from build123d import *

# Parameters (mm, degrees)
SKETCH1_W           = 100
SKETCH1_H           = 100
BOSS_EXTRUDE1_DEPTH = 2
BOSS_EXTRUDE2_DEPTH = 1
BOSS_EXTRUDE5_DEPTH = 1
SKETCH10_R          = 14.102334265
CUT_EXTRUDE1_DEPTH  = 1.5


with BuildPart() as part:
    # Sketch1 → Boss-Extrude1 (new body)
    with BuildSketch(Plane(origin=(0, 0, 0), x_dir=(1, 0, 0), z_dir=(0, 1, 0))):
        Rectangle(SKETCH1_W, SKETCH1_H)
    extrude(amount=BOSS_EXTRUDE1_DEPTH)

    # Inner Lines Incorrect → Boss-Extrude2 (add)
    with BuildSketch(Plane(origin=(0, 2, 0), x_dir=(-1, 0, 0), z_dir=(0, 1, 0))):
        with BuildLine():
            Line((-9.740714552, -37.307950056), (44.463704926, -38.16254763))
            Line((44.463704926, -38.16254763), (36.373030269, -23.4794714))
            Line((36.373030269, -23.4794714), (30.780994203, -23.4794714))
            Line((30.780994203, -23.4794714), (26.974802478, -16.868717352))
            ThreePointArc((26.974802478, -16.868717352), (-25.050764907, 33.390013397), (-9.740714552, -37.307950056))
        make_face()
    extrude(amount=BOSS_EXTRUDE2_DEPTH)

    # Perfect Trace FT Logo → Boss-Extrude5 (add)
    with BuildSketch(Plane(origin=(0, 3, 0), x_dir=(-1, 0, 0), z_dir=(0, 1, 0))):
        with BuildLine():
            Line((30.780994203, -23.4794714), (25.071735693, -13.56339083))
            Line((25.071735693, -13.56339083), (12.86572713, -13.582342535))
            ThreePointArc((12.86572713, -13.582342535), (-18.847428313, 21.043350665), (-3.934978039, -23.4794714))
            Line((-3.934978039, -23.4794714), (30.780994203, -23.4794714))
        make_face()
    extrude(amount=BOSS_EXTRUDE5_DEPTH)

    # Sketch10 → Cut-Extrude1 (cut)
    with BuildSketch(Plane(origin=(0, 4, 0), x_dir=(1, 0, 0), z_dir=(0, 1, 0))):
        with Locations(Location((6.665815692, -0.364658396, 0), (0, 0, 270))):
            Circle(SKETCH10_R)
    extrude(amount=-CUT_EXTRUDE1_DEPTH, mode=Mode.SUBTRACT)


solid = part.part
Work out the finished part from the listing and answer in its coordinate system (mm). A direction names the side the tool comes from. Coordinates: 2 decimals unless noted, no trailing zeros. Write each loop counter-clockwise with the first axis right and the second up, starting at its lowest first coordinate (ties: lowest second). Pieces come first, ordered by that corner, then holes.
1. The part is cut by section A-A, the plane x = 33.5. Write down the section's boundary in (y, z), and give its area (3 significant figures).
Results list:
outline: (0, -50) - (2, -50) - (2, -26.26) - (3, -26.26) - (3, 26.98) - (2, 26.98) - (2, 50) - (0, 50) - close
area: 253 mm2
2. For a pull along Z with two mould halves and no side action, classify faces 1 (the flat face through (-6, 4, -10)), 2 (the cylindrical face through (-1.915, 3.26, -10.826)), 3 (the flat face through (-40.475, 2.493, -30.924)) as +Z half, -Z half, draft (parallel to the pull), parting line (faces both ways), or undercut.
Results list:
face 1: draft
face 2: undercut
face 3: +Z half
3. The part is cut by section D-D, the plane x = -21. Write down the section's boundary in (y, z), and give its area (3 significant figures).
Results list:
outline: (0, -50) - (2, -50) - (2, -37.79) - (3, -37.79) - (3, -23.48) - (4, -23.48) - (4, -13.57) - (3, -13.57) - (3, 26.12) - (2, 26.12) - (2, 50) - (0, 50) - close
area: 274 mm2
4. Consider line 1 along Y through (x, z) = (18, 37); line 2 along Y through (x, z) = (-19.5, -37); line 3 along X through (y, z) = (3.7, 8). Determine where each line is inside the solid, lowest interval first.
Results list:
line 1: y = 0 to 2
line 2: y = 0 to 3
line 3: x = -16.09 to -5.19, 18.52 to 29.42
5. The part is cut by section B-B, the plane z = 5. Write down the section's boundary in (x, y), and give its area (3 significant figures).
Results list:
outline: (-50, 0) - (50, 0) - (50, 2) - (44.18, 2) - (44.18, 3) - (30.21, 3) - (30.21, 4) - (19.98, 4) - (19.98, 2.5) - (-6.65, 2.5) - (-6.65, 4) - (-16.88, 4) - (-16.88, 3) - (-30.85, 3) - (-30.85, 2) - (-50, 2) - close
area: 282 mm2
6. The part is cut by section C-C, the plane z = 29.5. Write down the section's boundary in (x, y), and give its area (3 significant figures).
Results list:
outline: (-50, 0) - (50, 0) - (50, 2) - (30.75, 2) - (30.75, 3) - (-17.41, 3) - (-17.41, 2) - (-50, 2) - close
area: 248 mm2
7. Flat-ended cylindrical pins translate along their axes: pin 1 (0.8 mm diameter, centred on x = -32.5, y = 2.5, fed in from +Z); pin 2 (0.8 mm diameter, centred on x = -16, y = 3.5, fed in from -Z); pin 3 (22.5 mm diameter, centred on x = 6.67, z = 0.36, fed in from +Y); pin 4 (1 mm diameter, centred on x = -21.5, z = 19, fed in from -Y). Find the tip coordinate at first contact, or state that the pin passes through.
Results list:
pin 1: stops at z = -23.48
pin 2: stops at z = -23.48
pin 3: stops at y = 2.5
pin 4: stops at y = 0
8. For faces 4 (the flat face through (-1, 0, -1)), 5 (the flat face through (7, 2.5, 0)), determine the directions among +Z, -Z, +X, -X, +Y, -Y from which every point of the face is accessible in a straight line to the end or side of a thin tool.
Results list:
face 4: +Z, -Z, +X, -X, -Y
face 5: +Y
